Part model, mm, in its own coordinate system. A direction names the side the tool comes from. Coordinates: 2 decimals unless noted, no trailing zeros. Loops run counter-clockwise (first coordinate to the right, second up) from the corner with the lowest first, then second, coordinate; pieces in that order, holes last. Notation, with made-up numbers: M -15,-18 L 22,-18 A36 cw 22,19 Z; hole C 64,28 d7. An arc over 180 degrees is marked long. Answer as a JSON object with one key per item and string values. Group by question number.
1. Mould opens along X. For faces 1 (the face through (14.93, -17.88, -49.8)), 2 (the face through (20, -25, 1)), 3 (the face through (-61.536, 1.302, -22.414)) say: released by +X, released by -X, zero draft, split by the parting line, or undercut.
2. Saw through at D-D on z = -55.5. Write the cut outline in (x, y).
3. 3-axis set-ups, long thin cutter, end or side, ignore diameter. For faces 4 (the face through (-93, 15, -10)), 5 (the face through (25, -15, 1)), 6 (the face through (-33, -18, -10)), 7 (the face through (-109, 10, 1)): which of +Z, -Z, +X, -X, +Y, -Y reach the whole face in a straight line?
4. Drill centre lines: L1, parallel to X at y = -22.25, z = 0; L2, parallel to Y at x = -17, z = 41.5; L3, parallel to Z at x = 76.5, y = -17.25. Where is each one in solid material? Low to high.
5. Saw through at C-C on x = 76.5. Write the cut outline in (y, z).
6. Saw through at A-A on z = 0. Write the cut outline in (x, y).
7. Drop flat-ended pins along their axis: pin 1 Ø5 at (y, z) = (-17.5, -1) entering from -X; pin 2 Ø12 at (y, z) = (9.5, 26) entering from -X; pin 3 Ø6 at (x, y) = (61.5, -14.5) entering from +Z. Give the stop position or say it passes through.
8. Saw through at B-B on y = -4. Write the cut outline in (x, z).
from build123d import *
from build123d import SkipClean  # not in build123d's __all__

# Parameters (mm, degrees)
F0_R     = 22.5
F1_DEPTH = 25
F2_DEPTH = 20
F4_START = 63.501
F4_DEPTH = 127.002


with BuildPart() as f1:
    # F0 (on Front) → F1 (new body)
    with BuildSketch(Plane.XZ):
        with BuildLine():
            ThreePointArc((-51.7071428571, -62.3953405344), (-14.6067671933, -40.5179193162), (0, 0))
            ThreePointArc((0, 0), (-14.6067671933, 40.5179193162), (-51.7071428571, 62.3953405344))
            ThreePointArc((-51.7071428571, 62.3953405344), (-127, 0), (-51.7071428571, -62.3953405344))
        make_face()
        with BuildLine():
            ThreePointArc((-83.6556443707, 10), (-63.5, 22.5), (-43.3443556293, 10))
            Line((-43.3443556293, 10), (-23.5, 10))
            Line((-23.5, 10), (-23.5, -10))
            Line((-23.5, -10), (-43.3443556293, -10))
            ThreePointArc((-43.3443556293, -10), (-63.5, -22.5), (-83.6556443707, -10))
            Line((-83.6556443707, -10), (-103.5, -10))
            Line((-103.5, -10), (-103.5, 10))
            Line((-103.5, 10), (-83.6556443707, 10))
        make_face(mode=Mode.SUBTRACT)
        with BuildLine():
            ThreePointArc((-51.7071428571, 62.3953405344), (-14.6067671933, 40.5179193162), (0, 0))
            ThreePointArc((0, 0), (-14.6067671933, -40.5179193162), (-51.7071428571, -62.3953405344))
            Line((-51.7071428571, -62.3953405344), (83.4642857143, -36.8476420479))
            ThreePointArc((83.4642857143, -36.8476420479), (39, 0), (83.4642857143, 36.8476420479))
            Line((83.4642857143, 36.8476420479), (-51.7071428571, 62.3953405344))
        make_face()
        with BuildLine():
            ThreePointArc((114, 0), (105.3739563819, 23.927905108), (83.4642857143, 36.8476420479))
            ThreePointArc((83.4642857143, 36.8476420479), (39, 0), (83.4642857143, -36.8476420479))
            ThreePointArc((83.4642857143, -36.8476420479), (105.3739563819, -23.927905108), (114, 0))
        make_face()
        with Locations((76.5, 0)):
            Circle(F0_R, mode=Mode.SUBTRACT)
    extrude(amount=F1_DEPTH)

    # F0 (on Front) → F2 (join)
    with BuildSketch(Plane.XZ):
        with BuildLine():
            ThreePointArc((-51.7071428571, -62.3953405344), (-14.6067671933, -40.5179193162), (0, 0))
            ThreePointArc((0, 0), (-14.6067671933, 40.5179193162), (-51.7071428571, 62.3953405344))
            ThreePointArc((-51.7071428571, 62.3953405344), (-127, 0), (-51.7071428571, -62.3953405344))
        make_face()
        with BuildLine():
            ThreePointArc((-83.6556443707, 10), (-63.5, 22.5), (-43.3443556293, 10))
            Line((-43.3443556293, 10), (-23.5, 10))
            Line((-23.5, 10), (-23.5, -10))
            Line((-23.5, -10), (-43.3443556293, -10))
            ThreePointArc((-43.3443556293, -10), (-63.5, -22.5), (-83.6556443707, -10))
            Line((-83.6556443707, -10), (-103.5, -10))
            Line((-103.5, -10), (-103.5, 10))
            Line((-103.5, 10), (-83.6556443707, 10))
        make_face(mode=Mode.SUBTRACT)
    with SkipClean():  # cleaning this boolean's faces spoils the solid; the shape is the same uncleaned
        extrude(amount=-F2_DEPTH)

    # F3 (on Top) → F4 (intersect)
    with BuildSketch(Plane.XY.offset(F4_START)):
        Polygon((-75.3271334507, 20), (-158.5341542959, 20), (-158.5341542959, 10), (-78.9921499119, 10), (-37.6571663732, -25), (141.5535062551, -25), (141.5535062551, -15), (-33.9921499119, -15), align=None)
    with SkipClean():  # cleaning this boolean's faces spoils the solid; the shape is the same uncleaned
        extrude(amount=-F4_DEPTH, mode=Mode.INTERSECT)


solid = f1.part
Outcome:
{
 "1": {"face 1": "released by +X", "face 2": "zero draft", "face 3": "undercut"},
 "2": {"outline": "M -94.35,10 L -78.99,10 L -37.66,-25 L -15.22,-25 L -15.22,-15 L -33.99,-15 L -75.33,20 L -94.35,20 Z"},
 "3": {"face 4": "+X, +Y, -Y", "face 5": "+Z, -Z, +X, +Y", "face 6": "-X, +Y, -Y", "face 7": "+Z, -Z, -X, -Y"},
 "4": {"L1": "x = -23.5 to 54, 99 to 114", "L2": "y = -25 to -15", "L3": "z = -38.16 to -22.5, 22.5 to 38.16"},
 "5": {"outline": "M -25,-38.16 L -15,-38.16 L -15,-22.5 L -25,-22.5 Z; M -25,22.5 L -15,22.5 L -15,38.16 L -25,38.16 Z"},
 "6": {"outline": "M -127,10 L -103.5,10 L -103.5,20 L -127,20 Z; M -23.5,-25 L 54,-25 L 54,-15 L -23.5,-15 Z; M 99,-25 L 114,-25 L 114,-15 L 99,-15 Z"},
 "7": {"pin 1": "stops at x = -23.5", "pin 2": "stops at x = -123.76", "pin 3": "stops at z = 41.56"},
 "8": {"outline": "M -62.46,-63.49 A63.5 ccw -51.71,-62.4 L -46.98,-61.5 L -46.98,-15.28 A22.5 cw -62.46,-22.48 Z; M -62.46,22.48 A22.5 cw -46.98,15.28 L -46.98,61.5 L -51.71,62.4 A63.5 ccw -62.46,63.49 Z"}
}
